```python
from build123d import *

# Parameters (mm, degrees)
F0_R     = 10.15
F0_R_2   = 8.95
F1_DEPTH = 71
F0_R_3   = 6.95
F2_DEPTH = 2
F4_DEPTH = 20
F5_DEPTH = 2


with BuildPart() as f1:
    # F0 (on Top) → F1 (new body)
    with BuildSketch(Plane.XY):
        Circle(F0_R)
        Circle(F0_R_2, mode=Mode.SUBTRACT)
    extrude(amount=F1_DEPTH)

    # F0 (on Top) → F2 (join)
    with BuildSketch(Plane.XY):
        Circle(F0_R_2)
        Circle(F0_R_3, mode=Mode.SUBTRACT)
    extrude(amount=F2_DEPTH)

    # F3 (on face) → F4 (cut)
    with BuildSketch(Plane.XY.offset(71)):
        with BuildLine():
            Line((-8.5937477273, 2.5), (-9.8373014592, 2.5))
            ThreePointArc((-9.8373014592, 2.5), (-9.8973111438, 2.2507181348), (-9.9510049744, 2))
            Line((-9.9510049744, 2), (-8.7236746844, 2))
            ThreePointArc((-8.7236746844, 2), (-8.6623195362, 2.2509376388), (-8.5937477273, 2.5))
        make_face()
        with BuildLine():
            ThreePointArc((-9.9510049744, -2), (-9.8973111438, -2.2507181348), (-9.8373014592, -2.5))
            Line((-9.8373014592, -2.5), (-8.5937477273, -2.5))
            ThreePointArc((-8.5937477273, -2.5), (-8.6623195362, -2.2509376388), (-8.7236746844, -2))
            Line((-8.7236746844, -2), (-9.9510049744, -2))
        make_face()
        with BuildLine():
            Line((8.7236746844, 2), (9.9510049744, 2))
            ThreePointArc((9.9510049744, 2), (9.8973111438, 2.2507181348), (9.8373014592, 2.5))
            Line((9.8373014592, 2.5), (8.5937477273, 2.5))
            ThreePointArc((8.5937477273, 2.5), (8.6623195362, 2.2509376388), (8.7236746844, 2))
        make_face()
        with BuildLine():
            ThreePointArc((9.8373014592, -2.5), (9.8973111438, -2.2507181348), (9.9510049744, -2))
            Line((9.9510049744, -2), (8.7236746844, -2))
            ThreePointArc((8.7236746844, -2), (8.6623195362, -2.2509376388), (8.5937477273, -2.5))
            Line((8.5937477273, -2.5), (9.8373014592, -2.5))
        make_face()
    extrude(amount=-F4_DEPTH, mode=Mode.SUBTRACT)

    # F3 (on face) → F5 (join)
    with BuildSketch(Plane.XY.offset(71)):
        with BuildLine():
            Line((-7.1543120913, 2), (-8.7236746844, 2))
            ThreePointArc((-8.7236746844, 2), (-8.95, 0), (-8.7236746844, -2))
            Line((-8.7236746844, -2), (-7.1543120913, -2))
            Line((-7.1543120913, -2), (-7.1543120913, 2))
        make_face()
        with BuildLine():
            Line((-8.7236746844, 2), (-9.9510049744, 2))
            ThreePointArc((-9.9510049744, 2), (-10.15, 0), (-9.9510049744, -2))
            Line((-9.9510049744, -2), (-8.7236746844, -2))
            ThreePointArc((-8.7236746844, -2), (-8.95, 0), (-8.7236746844, 2))
        make_face()
        with BuildLine():
            ThreePointArc((8.95, 0), (8.8932386796, 1.0063825252), (8.7236746844, 2))
            Line((8.7236746844, 2), (7.1543120913, 2))
            Line((7.1543120913, 2), (7.1543120913, -2))
            Line((7.1543120913, -2), (8.7236746844, -2))
            ThreePointArc((8.7236746844, -2), (8.8932386796, -1.0063825252), (8.95, 0))
        make_face()
        with BuildLine():
            ThreePointArc((9.9510049744, -2), (10.1001287242, -1.0049376872), (10.15, 0))
            ThreePointArc((10.15, 0), (10.1001287242, 1.0049376872), (9.9510049744, 2))
            Line((9.9510049744, 2), (8.7236746844, 2))
            ThreePointArc((8.7236746844, 2), (8.8932386796, 1.0063825252), (8.95, 0))
            ThreePointArc((8.95, 0), (8.8932386796, -1.0063825252), (8.7236746844, -2))
            Line((8.7236746844, -2), (9.9510049744, -2))
        make_face()
    extrude(amount=F5_DEPTH)


solid = f1.part
```
Geometry: final body of the model. Coordinates: model frame, mm. A direction names the side the tool comes from. Round coordinates to 2 decimals unless told otherwise and drop trailing zeros. Write each loop counter-clockwise with the first axis right and the second up, starting at its lowest first coordinate (ties: lowest second). Pieces come first, ordered by that corner, then holes. Notation, with made-up numbers: (42.5, 75.25) -> (46.5, 75.25) arc R21 cw to (46.5, 97.25) -> close; hole circle Ø1 at (0, -23). An arc over 180 degrees is marked (long way). Return JSON: item names as keys, results as strings.
Q1. Section B-B on y = 4.5. Return the cut outline in (x, z).
From the geometry:
{"outline": "(-9.1, 0) -> (-5.3, 0) -> (-5.3, 2) -> (-7.74, 2) -> (-7.74, 71) -> (-9.1, 71) -> close; (5.3, 0) -> (9.1, 0) -> (9.1, 71) -> (7.74, 71) -> (7.74, 2) -> (5.3, 2) -> close"}
Q2. First-contact query: pin 1 Ø0.6 at (x, z) = (-9, 62) entering from +Y; pin 2 Ø1.5 at (x, z) = (-6.5, 55) entering from -Y; pin 3 Ø1 at (x, z) = (9.5, 61) entering from -Y. Flat tips, straight axial feed; report the tip coordinate or a pass-through.
From the geometry:
{"pin 1": "y = 5.23", "pin 2": "y = -8.36", "pin 3": "y = -4.69"}
Q3. Section C-C on z = 38. Return the cut outline in (x, y).
From the geometry:
{"outline": "circle Ø20.3 at (0, 0); hole circle Ø17.9 at (0, 0)"}
Q4. Ray query, line 1 (Y direction, x = 0, z = 45); line 2 (X direction, y = 0.5, z = 31.5); line 3 (X direction, y = 5, z = 3). Return the intervals inside material, ascending.
From the geometry:
{"line 1": "-10.15 to -8.95, 8.95 to 10.15", "line 2": "-10.14 to -8.94, 8.94 to 10.14", "line 3": "-8.83 to -7.42, 7.42 to 8.83"}
Q5. Section A-A on x = 0. Return the cut outline in (y, z).
From the geometry:
{"outline": "(-10.15, 0) -> (-6.95, 0) -> (-6.95, 2) -> (-8.95, 2) -> (-8.95, 71) -> (-10.15, 71) -> close; (6.95, 0) -> (10.15, 0) -> (10.15, 71) -> (8.95, 71) -> (8.95, 2) -> (6.95, 2) -> close"}
Q6. Set-up query: faces 4 (the flat face through (8, 0, 71)), 5 (the flat face through (0, 9.2, 71)), 6 (the flat face through (0, -9.1, 71)), 7 (the flat face through (9, 2.5, 61)). Return all of +Z, -Z, +X, -X, +Y, -Y with unobstructed straight access to the full face (end or side cutting, diameter ignored); none if empty.
From the geometry:
{"face 4": "none", "face 5": "+Z, +X, -X, +Y", "face 6": "+Z, +X, -X, -Y", "face 7": "+Z, +X, -X"}
Q7. Mould query, pull axis Y, two halves, no side actions, for faces 1 (the flat face through (0, -7.3, 2)), 2 (the flat face through (7.154, 0, 72)), 3 (the flat face through (-9, -2, 62)). Classes: +Y half, -Y half, draft (parallel to the pull), parting line (faces both ways), or undercut.
From the geometry:
{"face 1": "undercut", "face 2": "draft", "face 3": "undercut"}
